Can you work these out from the model? Positions are in its coordinate system, mm. Face numbers are marked on the shaded views. A direction names the side the tool comes from. Coordinates: 2 decimals unless noted, no trailing zeros. Order: outer loops, then holes, each group sorted by start corner. A loop starts at its lowest first (then second) coordinate and runs counter-clockwise, first axis right, second up. Notation, with made-up numbers: (-31.5, -11.5) -> (-7.5, -11.5) arc R34 ccw to (-7.5, 21.5) -> close; hole circle Ø6 at (59, 11.5). An arc over 180 degrees is marked (long way). Write item = value, one per line.
```python
from build123d import *

# Parameters (mm, degrees)
F0_R     = 4
F1_DEPTH = 3
F2_DEPTH = 9
F3_R     = 1.5
F4_DEPTH = 3


with BuildPart() as f1:
    # F0 (on Top) → F1 (new body)
    with BuildSketch(Plane.XY):
        Polygon((0, 41), (0, 0), (42.5, 0), (42.5, 31), (32.5, 31), (32.5, 41), align=None)
        with Locations((8, 8)):
            Circle(F0_R, mode=Mode.SUBTRACT)
        with Locations((8, 8)):
            Circle(F0_R)
    extrude(amount=-F1_DEPTH)

    # F0 (on Top) → F2 (join)
    with BuildSketch(Plane.XY):
        with Locations((8, 8)):
            Circle(F0_R)
    extrude(amount=F2_DEPTH)

    # F3 (on face) → F4 (join)
    with BuildSketch(Plane.XY.offset(9)):
        with Locations((8, 8)):
            Circle(F3_R)
    extrude(amount=F4_DEPTH)


solid = f1.part
```
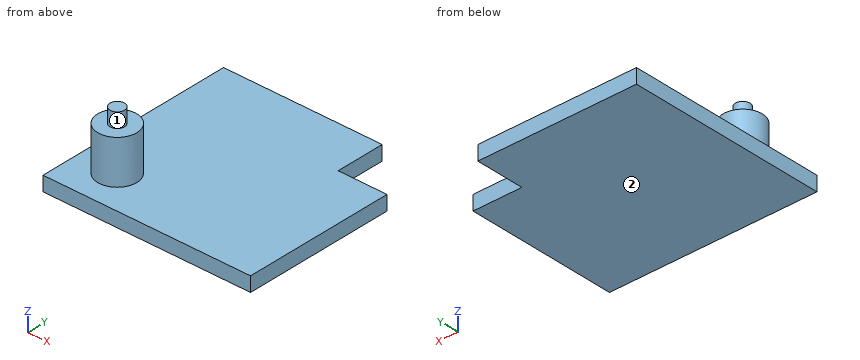
Item 1: I want a section at A-A, the plane x = 8. Please give me the cut outline in (y, z).
A:
outline = (0, -3) -> (41, -3) -> (41, 0) -> (12, 0) -> (12, 9) -> (9.5, 9) -> (9.5, 12) -> (6.5, 12) -> (6.5, 9) -> (4, 9) -> (4, 0) -> (0, 0) -> close
Item 2: If I drill on probe 1 along Z at (x, y) = (34.5, 25); probe 2 along Y at (x, z) = (8.5, 5.5); probe 3 along X at (y, z) = (7, 8.5), over which ranges is the centre line in solid material (lowest first)?
A:
probe_1 = -3 to 0
probe_2 = 4.03 to 11.97
probe_3 = 4.13 to 11.87
Item 3: I want a section at D-D, the plane y = 29. Please give me the cut outline in (x, z), plus the area to 4 significant figures.
A:
outline = (0, -3) -> (42.5, -3) -> (42.5, 0) -> (0, 0) -> close
area = 127.5 mm2
Item 4: I'm going to push flat-ended pins straight in: P1, Ø2, axis at x = 12, y = 16.5, coming from the +Z side; P2, Ø12, axis at x = 5, y = 15, coming from the +Z side; P3, Ø3.5, axis at x = 35, z = -1, coming from the +Y side; P4, Ø4, axis at x = 8.5, y = 10, coming from the +Z side. Where does each tip first touch, or does it pass through?
A:
P1 = 0
P2 = 9
P3 = 31
P4 = 12
Item 5: For the marked faces 1 and 2, which set-ups out of +Z, -Z, +X, -X, +Y, -Y let a thin tool reach every point of the face, with its end or its side?
A:
face_1 = +Z
face_2 = -Z, +X, -X, +Y, -Y
Item 6: I want a section at C-C, the plane z = -1. Please give me the cut outline in (x, y), plus the area to 3 significant figures.
A:
outline = (0, 0) -> (42.5, 0) -> (42.5, 31) -> (32.5, 31) -> (32.5, 41) -> (0, 41) -> close
area = 1,640 mm2
Item 7: I want a section at B-B, the plane y = 8. Please give me the cut outline in (x, z), plus the area to 4 significant figures.
A:
outline = (0, -3) -> (42.5, -3) -> (42.5, 0) -> (12, 0) -> (12, 9) -> (9.5, 9) -> (9.5, 12) -> (6.5, 12) -> (6.5, 9) -> (4, 9) -> (4, 0) -> (0, 0) -> close
area = 208.5 mm2
